Can you work these out from the model? Positions are in its coordinate system, mm. A direction names the side the tool comes from. Give positions to 0.01 mm unless a question says otherwise; leave off trailing zeros. Order: outer loops, then holes, each group sorted by start corner. A loop starts at its lowest first (then second) coordinate and runs counter-clockwise, first axis right, second up. Notation, with made-up numbers: M -8.5,34 L 20.5,34 A8 cw 20.5,43 Z; hole C -17.75,44 d1. An arc over 180 degrees is marked long. Use a Markdown table: item, result. Add a question column.
from build123d import *

# Parameters (mm, degrees)
SKETCH1_W           = 250
SKETCH1_H           = 300
BOSS_EXTRUDE1_DEPTH = 350
SKETCH2_R           = 14.75
BOSS_EXTRUDE2_DEPTH = 10
LPATTERN2_COUNT     = 2
LPATTERN2_PITCH     = 260


with BuildPart() as part:
    # Sketch1 → Boss-Extrude1 (new body)
    with BuildSketch(Plane(origin=(0, 0, 0), x_dir=(1, 0, 0), z_dir=(0, 1, 0))):
        with Locations((-29.444356891, 74.84242821)):
            Rectangle(SKETCH1_W, SKETCH1_H)
    extrude(amount=BOSS_EXTRUDE1_DEPTH)

    # Sketch2 → Boss-Extrude2 (add)
    with BuildSketch(Plane(origin=(95.555643109, 0, 0), x_dir=(0, 0, -1), z_dir=(1, 0, 0))):
        with Locations((-75.15757179, 0)):
            Circle(SKETCH2_R)
        with Locations(Location((224.84242821, 0, 0), (0, 0, 180))):
            Circle(SKETCH2_R)
    boss_extrude2 = extrude(amount=BOSS_EXTRUDE2_DEPTH)

    # LPattern2: Boss-Extrude2 ×2
    with Locations(*[(-i * LPATTERN2_PITCH, 0, 0) for i in range(1, LPATTERN2_COUNT)]):
        add(boss_extrude2)


solid = part.part
1. Will these pins go through, and if not, where does the flat tip stop? pin 1 (1 mm diameter, centred on x = -103.5, z = -86.5, fed in from -Y); pin 2 (6 mm diameter, centred on x = -41, y = 94, fed in from +Z); pin 3 (8 mm diameter, centred on y = 233, z = -193.5, fed in from +X).
2. On a 3-axis mill with a long thin cutter (end or side, diameter ignored), from which of +Z, -Z, +X, -X, +Y, -Y can I reach the whole of each face in a straight line? I mean faces 1 (the face through (-159.514, -5.649, 61.532)), 2 (the face through (-164.444, 0, 75)), 3 (the face through (95.556, -3, 79)), 4 (the face through (95.556, 0, -225)), 5 (the face through (100.486, -5.649, 61.532)). Say none if no direction works.
3. I need wall thicknesses on L1, parallel to Z at x = 86, y = 85.5; L2, parallel to Y at x = 8, z = -73.5; L3, parallel to X at y = 326, z = 48. Which ranges of each line are inside material? Lowest first, please. Write a range as [from, to].
4. We'd pull the mould along Z, two halves only. Please class faces 6 (the face through (-159.51, -0.65, -239.58)), 7 (the face through (-31, 173, 75.158)), 8 (the face through (-31, 173, -224.842)), 9 (the face through (-154.444, 0, -225)): +Z half, -Z half, draft (parallel to the pull), parting line (faces both ways), or undercut.
5. If we section it at A-A, the plane z = 2: List the corners of the cut face in (x, y) for me.
6. If we section it at B-B, the plane x = -22: List the corners of the cut face in (y, z) for me.
Geometry results:
| question | item | result |
|---|---|---|
| 1 | pin 1 | stops at y = 0 |
| 1 | pin 2 | stops at z = 75.16 |
| 1 | pin 3 | stops at x = 95.56 |
| 2 | face 1 | -X |
| 2 | face 2 | +Z, -Z, -X, +Y, -Y |
| 2 | face 3 | +Z, -Y |
| 2 | face 4 | -Z, -Y |
| 2 | face 5 | +X |
| 3 | L1 | z = [-224.84, 75.16] |
| 3 | L2 | y = [0, 350] |
| 3 | L3 | x = [-154.44, 95.56] |
| 4 | face 6 | undercut |
| 4 | face 7 | +Z half |
| 4 | face 8 | -Z half |
| 4 | face 9 | draft |
| 5 | outline | M -154.44,0 L 95.56,0 L 95.56,350 L -154.44,350 Z |
| 6 | outline | M 0,-224.84 L 350,-224.84 L 350,75.16 L 0,75.16 Z |
